Solid Edge part; units mm, degrees
sketch "Sketch1" plane through (0, 0, 0) normal (0, -1, 0) x (1, 0, 0)
  line L0 (37.5, 21.6506) -> (0, 43.3013)
  line L1 (0, 43.3013) -> (-37.5, 21.6506)
  line L2 (-37.5, 21.6506) -> (-37.5, -21.6506)
  line L3 (-37.5, -21.6506) -> (0, -43.3013)
  line L4 (0, -43.3013) -> (37.5, -21.6506)
  line L5 (37.5, -21.6506) -> (37.5, 21.6506)
  dimension "D1" = 37.5
extrude "Protrusion1" add sketch "Sketch1" against normal blind 20
sketch "Sketch2" plane through (0, 20, 0) normal (0, 1, 0) x (-0.866, 0, 0.5)
  circle A0 centre (0, 0) radius 15.5
extrude "ExtrudedCutout_1" cut sketch "Sketch2" against normal blind 146.9275
hole "Hole_1" at (0, 20, 0) direction (0, -1, 0) diameter 42.587 depth 15 thread major 48 thread length 2
Verification items for the finished model (mm, model axes). A direction names the side the tool comes from. Round coordinates to 2 decimals unless told otherwise and drop trailing zeros. Write each loop counter-clockwise with the first axis right and the second up, starting at its lowest first coordinate (ties: lowest second). Pieces come first, ordered by that corner, then holes. Notation, with made-up numbers: (-34.75, -17.5) -> (-9.75, -17.5) arc R30 cw to (-9.75, 11.5) -> close; hole circle Ø5 at (-13.75, 88). An arc over 180 degrees is marked (long way). Write each question's results on one line, items separated by ' | '.
Q1. Sectioned sample at C-C, the plane x = 4. Record the boundary of the cut face in (y, z).
Derived:
outline: (0, -40.99) -> (20, -40.99) -> (20, -20.91) -> (5, -20.91) -> (5, -14.97) -> (0, -14.97) -> close; (0, 14.97) -> (5, 14.97) -> (5, 20.91) -> (20, 20.91) -> (20, 40.99) -> (0, 40.99) -> close
Q2. Sectioned sample at A-A, the plane z = 0. Record the boundary of the cut face in (x, y), and give its area (3 significant figures).
Derived:
outline: (-37.5, 0) -> (-15.5, 0) -> (-15.5, 5) -> (-21.29, 5) -> (-21.29, 20) -> (-37.5, 20) -> close; (15.5, 0) -> (37.5, 0) -> (37.5, 20) -> (21.29, 20) -> (21.29, 5) -> (15.5, 5) -> close | area: 706 mm²
Q3. Thickness scan on probe 1 along X at (y, z) = (3.8, 0); probe 2 along Z at (x, y) = (0, 10); probe 3 along X at (y, z) = (9, 0). Record the ranges inside material, lowest first.
Derived:
probe 1: x = -37.5 to -15.5, 15.5 to 37.5 | probe 2: z = -43.3 to -21.29, 21.29 to 43.3 | probe 3: x = -37.5 to -21.29, 21.29 to 37.5
Q4. Sectioned sample at B-B, the plane y = 6.5. Record the boundary of the cut face in (x, z), and give its area (3 significant figures).
Derived:
outline: (-37.5, -21.65) -> (0, -43.3) -> (37.5, -21.65) -> (37.5, 21.65) -> (0, 43.3) -> (-37.5, 21.65) -> close; hole circle Ø42.59 at (0, 0) | area: 3,450 mm²
Q5. Go/stop test with flat-tipped pins: pin 1 Ø12 at (x, y) = (9, 12) entering from -Z; pin 2 Ø13 at (x, z) = (6.5, 3) entering from +Y; pin 3 Ø1 at (x, y) = (-22.5, 15.5) entering from -Z; pin 4 Ø12 at (y, z) = (9, 28.5) entering from +X. Record where each tip stops, or that it passes through.
Derived:
pin 1: stops at z = -41.57 | pin 2: passes through | pin 3: stops at z = -30.6 | pin 4: stops at x = 36.03
Q6. Sectioned sample at D-D, the plane x = 23. Record the boundary of the cut face in (y, z).
Derived:
outline: (0, -30.02) -> (20, -30.02) -> (20, 30.02) -> (0, 30.02) -> close
Q7. Draft check along Z on faces 1 (the face through (1, 0, -19)), 2 (the face through (19.012, 9.86, 32.324)), 3 (the face through (16, 5, 1)). Enter one of: released by +Z, released by -Z, zero draft, split by the parting line, or undercut.
Derived:
face 1: zero draft | face 2: released by +Z | face 3: undercut
Q8. Access from +Z, -Z, +X, -X, +Y, -Y to the whole of each face (thin tool, end or side, straight path). Record for faces 4 (the face through (-18.488, 9.86, 32.628)), 5 (the face through (20.787, 12.395, -4.616)).
Derived:
face 4: +Z, -X, +Y, -Y | face 5: +Y
